Model file for the job. Use its own axes, mm. Face numbers are marked on the shaded views. A direction names the side the tool comes from. Give positions to 0.01 mm unless a question says otherwise; leave off trailing zeros. Write each loop counter-clockwise with the first axis right and the second up, starting at its lowest first coordinate (ties: lowest second). Pieces come first, ordered by that corner, then holes. Notation, with made-up numbers: (-28.5, 75) - (-16.5, 75) arc R22 cw to (-16.5, 112) - close; hole circle Ø5 at (-8, -2). An arc over 180 degrees is marked (long way). Use a Markdown table: item, result. Add a question column.
```python
from build123d import *

# Parameters (mm, degrees)
SKETCH2_R          = 41.275
CUT_EXTRUDE1_DEPTH = 9.525


with BuildPart() as part:
    # Sketch1 → Revolve1 (revolve)
    with BuildSketch(Plane.XY):
        Polygon((0, 0), (-50.8, 0), (-50.8, -3.175), (-44.45, -3.175), (-44.45, -12.7), (0, -12.7), align=None)
    revolve(axis=Axis((0, -12.7, 0), (0, 1, 0)))

    # Sketch2 → Cut-Extrude1 (cut)
    with BuildSketch(Plane.XZ.offset(12.7)):
        Circle(SKETCH2_R)
    extrude(amount=-CUT_EXTRUDE1_DEPTH, mode=Mode.SUBTRACT)


solid = part.part
```
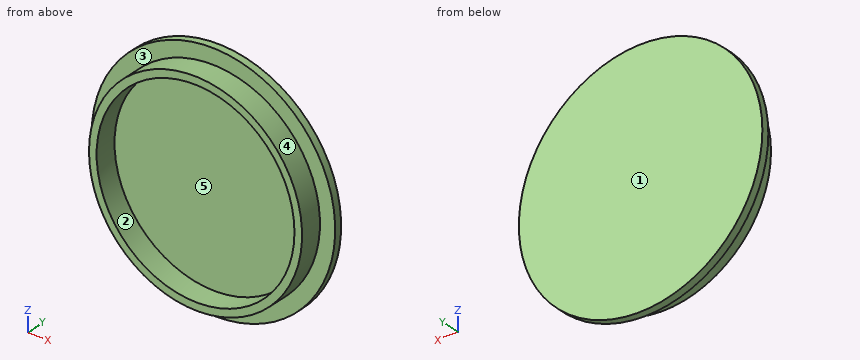
(1) Flat gauge pins, fed straight in: pin 1 (2 mm diameter, centred on x = 34.5, y = -8.5, fed in from -Z); pin 2 (5 mm diameter, centred on x = 37.5, y = -11, fed in from +Z); pin 3 (1 mm diameter, centred on x = 31, z = 7, fed in from +Y); pin 4 (1.5 mm diameter, centred on y = -9, z = -37.5, fed in from -X). Where does each tip first touch, or does it go through?
(2) Band-saw the part on D-D (z = -43). Write the cut outline in (x, y) (3 decimals), then the cut area to 3 significant figures.
(3) Two-plate mould, pull along X, no slides. Class the marked faces 3, 4 and 5: +X half, -X half, draft (parallel to the pull), parting line (faces both ways), or undercut.
(4) Band-saw the part on B-B (x = 0). Write the cut outline in (y, z) (3 decimals), then the cut area to 3 significant figures.
(5) Band-saw the part on C-C (y = -2). Write the cut outline in (x, z), then the cut area to 3 significant figures.
(6) Probe probe 1 along Z at (x, y) = (0, -10) (3 decimals); probe 2 along Y at (x, z) = (18.5, 26) (3 decimals); probe 3 along Z at (x, y) = (-24.5, -5). List the from-to ranges inside material, lowest first. Write a range as [from, to].
(7) Band-saw the part on A-A (z = 0). Write the cut outline in (x, y) (3 decimals).
(8) Which spindle directions (+Z, -Z, +X, -X, +Y, -Y) get a long thin tool onto all of the face, cutting with end or side? Do the marked faces 1 and 2. Say none if no direction does.
Model answer:
| question | item | result |
|---|---|---|
| 1 | pin 1 | stops at z = -29.22 |
| 1 | pin 2 | stops at z = 27.4 |
| 1 | pin 3 | stops at y = 0 |
| 1 | pin 4 | stops at x = -25 |
| 2 | outline | (-27.049, -3.175) - (-11.261, -3.175) - (-11.261, -12.7) - (11.261, -12.7) - (11.261, -3.175) - (27.049, -3.175) - (27.049, 0) - (-27.049, 0) - close |
| 2 | area | 386 mm^2 |
| 3 | face 3 | draft |
| 3 | face 4 | parting line |
| 3 | face 5 | undercut |
| 4 | outline | (-12.7, -44.45) - (-3.175, -44.45) - (-3.175, -50.8) - (0, -50.8) - (0, 50.8) - (-3.175, 50.8) - (-3.175, 44.45) - (-12.7, 44.45) - (-12.7, 41.275) - (-3.175, 41.275) - (-3.175, -41.275) - (-12.7, -41.275) - close |
| 4 | area | 383 mm^2 |
| 5 | outline | circle Ø101.6 at (0, 0) |
| 5 | area | 8,110 mm^2 |
| 6 | probe 1 | z = [-44.45, -41.275], [41.275, 44.45] |
| 6 | probe 2 | y = [-3.175, 0] |
| 6 | probe 3 | z = [-37.09, -33.22], [33.22, 37.09] |
| 7 | outline | (-50.8, -3.175) - (-44.45, -3.175) - (-44.45, -12.7) - (-41.275, -12.7) - (-41.275, -3.175) - (41.275, -3.175) - (41.275, -12.7) - (44.45, -12.7) - (44.45, -3.175) - (50.8, -3.175) - (50.8, 0) - (-50.8, 0) - close |
| 8 | face 1 | +Z, -Z, +X, -X, +Y |
| 8 | face 2 | -Y |
